CAD build for the part. Positions are in the model's coordinates, mm. A direction names the side the tool comes from. Give positions to 0.01 mm unless a question says otherwise; leave off trailing zeros. Write each loop counter-clockwise with the first axis right and the second up, starting at its lowest first coordinate (ties: lowest second). Pieces come first, ordered by that corner, then holes. Notation, with made-up numbers: (56, 28.25) -> (89, 28.25) arc R24 cw to (89, 63.25) -> close; hole circle Ø2 at (-39, -5.75). An arc over 180 degrees is marked (long way). Answer in a Markdown table with one row per item. Add a question column.
```python
from build123d import *

# Parameters (mm, degrees)
CUT_EXTRUDE2_DEPTH      = 33.111212995
CUT_EXTRUDE2_DEPTH_BACK = 33.111212995
SKETCH2_R               = 1.75
SKETCH2_R_2             = 2


with BuildPart() as part:
    # Sketch1 → Revolve1 (revolve)
    with BuildSketch(Plane.XY, mode=Mode.PRIVATE) as revolve1_sk:
        with BuildLine():
            Line((10.5, 14), (7.5, 14))
            Line((7.5, 14), (7.5, 19.2))
            ThreePointArc((7.5, 19.2), (6.972792206, 20.472792206), (5.7, 21))
            Line((5.7, 21), (5.5, 21))
            Line((5.5, 21), (5.5, 19))
            Line((5.5, 19), (2, 19))
            Line((2, 19), (2, 21.2))
            Line((2, 21.2), (0, 21.2))
            Line((0, 21.2), (0, 0))
            Line((0, 0), (4, 0))
            Line((4, 0), (4, 9.55))
            Line((4, 9.55), (10.5, 9.55))
            Line((10.5, 9.55), (10.5, 9.75))
            Line((10.5, 9.75), (11.5, 9.75))
            Line((11.5, 9.75), (11.5, 11.75))
            Line((11.5, 11.75), (10.5, 11.75))
            Line((10.5, 11.75), (10.5, 14))
        make_face()
    revolve(revolve1_sk.sketch.rotate(Axis((0, 0, 0), (1, 0, 0)), 180), axis=Axis((0, 0, 0), (1, 0, 0)))

    # Sketch2 → Cut-Extrude2 (cut, two sides: drawn at the far end of the back side and taken through both)
    with BuildSketch(Plane(origin=(0, 0, 0), x_dir=(0, 0, -1), z_dir=(1, 0, 0)).offset(-CUT_EXTRUDE2_DEPTH_BACK)):
        Circle(SKETCH2_R)
        with Locations((0, -5)):
            Circle(SKETCH2_R_2)
        with Locations((-4.330127019, 2.5)):
            Circle(SKETCH2_R_2)
        with Locations((4.330127019, 2.5)):
            Circle(SKETCH2_R_2)
    extrude(amount=CUT_EXTRUDE2_DEPTH + CUT_EXTRUDE2_DEPTH_BACK, mode=Mode.SUBTRACT)


solid = part.part
```
Item 1: Slice it at C-C, the plane x = 4.75. List the corners of the cut face in (y, z).
Item 2: Mould opens along Z. For faces 1 (the face through (4, 2, 0)), 2 (the face through (7.5, 1.3, 14.1)), 3 (the face through (3.726, 4.119, 18.548)), 4 (the face through (2, -7, 0)) say: released by +Z, released by -Z, zero draft, split by the parting line, or undercut.
Item 3: Slice it at B-B, the plane x = 2.5. List the corners of the cut face in (y, z), then the cut area to 3 significant figures.
Item 4: Probe L1, parallel to Z at x = 5, y = 0; L2, parallel to Z at x = 2.05, y = 0; L3, parallel to Z at x = 1.05, y = 2.5. List the from-to ranges inside material, lowest first. Write a range as from..to.
Item 5: Slice it at D-D, the plane z = 0. State how many separate pieces and enclosed holes the cut face has, then the cut area to 3 significant figures.
Item 6: Which spindle directions (+Z, -Z, +X, -X, +Y, -Y) get a long thin tool onto all of the face, cutting with end or side? Do faces 5 (the face through (1.972, 1.283, 5.917)), 6 (the face through (5.5, 16, 11)), 7 (the face through (11.007, 1.269, -9.667)). Say none if no direction does.
Item 7: Drop flat-ended pins along their axis: pin 1 Ø5.5 at (y, z) = (4.5, 2) entering from +X; pin 2 Ø1 at (x, z) = (2, -17) entering from -Y; pin 3 Ø3 at (x, y) = (6.5, -16.5) entering from +Z. Give the stop position or say it passes through.
Answer key:
| question | item | result |
|---|---|---|
| 1 | outline | circle Ø38 at (0, 0); hole circle Ø19.1 at (0, 0) |
| 2 | face 1 | undercut |
| 2 | face 2 | zero draft |
| 2 | face 3 | split by the parting line |
| 2 | face 4 | undercut |
| 3 | outline | circle Ø38 at (0, 0); hole circle Ø4 at (-5, 0); hole circle Ø3.5 at (0, 0); hole circle Ø4 at (2.5, -4.33); hole circle Ø4 at (2.5, 4.33) |
| 3 | area | 1,090 mm² |
| 4 | L1 | z = -19..-9.55, 9.55..19 |
| 4 | L2 | z = -19..-1.75, 1.75..19 |
| 4 | L3 | z = -21.05..-6.33, -2.33..2.33, 6.33..21.05 |
| 5 | separate pieces | 3 |
| 5 | enclosed holes | 0 |
| 5 | area | 234 mm² |
| 6 | face 5 | +X, -X |
| 6 | face 6 | none |
| 6 | face 7 | +X |
| 7 | pin 1 | stops at x = 4 |
| 7 | pin 2 | stops at y = -13.31 |
| 7 | pin 3 | stops at z = 14.58 |
